Check sheet for the drawn part. Datum: minimum x, y, z corner. Units: mm. Coordinates: 2 decimals unless noted, no trailing zeros. Loops run counter-clockwise (first coordinate to the right, second up) from the corner with the lowest first, then second, coordinate; pieces in that order, holes last. Notation, with made-up numbers: (46.5, -3) - (101.5, -3) arc R19 cw to (101.5, 30) - close; hole circle Ø7 at (-9.5, 33.5). An arc over 180 degrees is marked (long way). Answer as a JSON object with one key per item and string values. Group by question number.
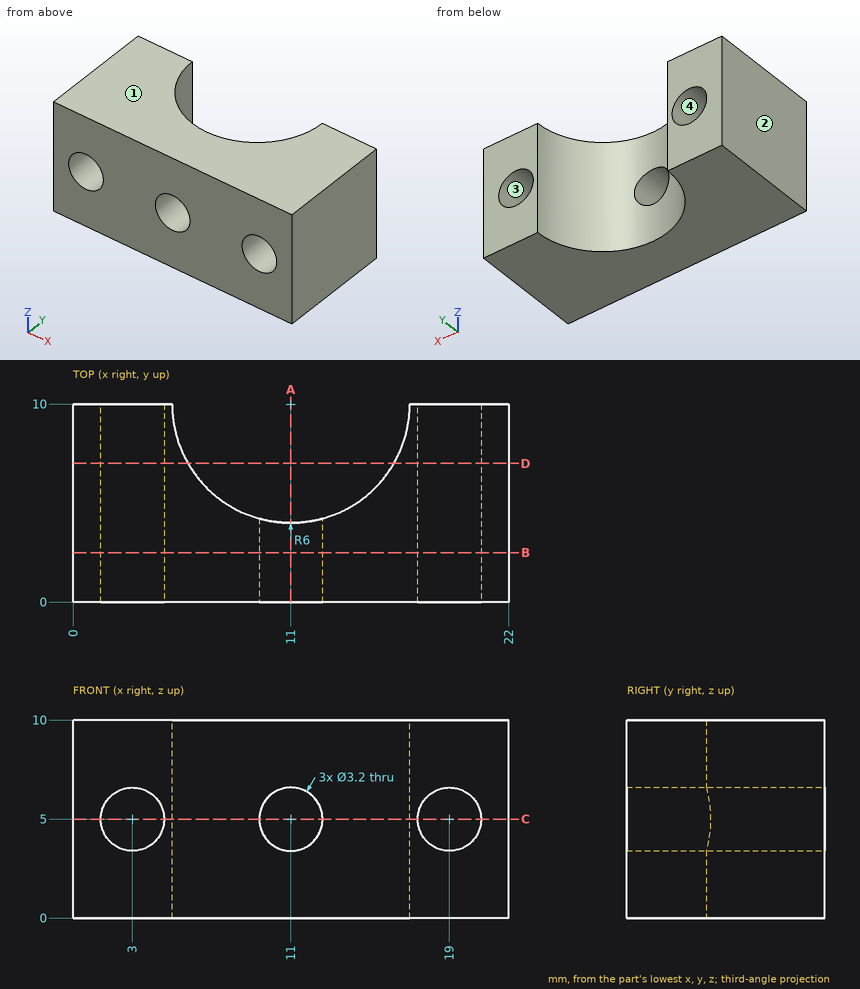
1. Sectioned sample at D-D on y = 7. Record the cut outline in (x, z), plus the area to 4 significant figures.
2. Gauge pin test, flat ends, axial feed: pin 1 (3 mm diameter, centred on x = 12, z = 7, fed in from +Y); pin 2 (1.9 mm diameter, centred on x = 11, z = 5, fed in from +Y). Record the tip position at first contact, or that the pin passes through.
3. Sectioned sample at C-C on z = 5. Record the cut outline in (x, y).
4. Release check for a two-part mould opening along Z. For the marked faces 1, 2, 3 and 4 record: released by +Z, released by -Z, zero draft, split by the parting line, or undercut.
5. Sectioned sample at B-B on y = 2.5. Record the cut outline in (x, z).
6. Sectioned sample at A-A on x = 11. Record the cut outline in (y, z).
7. Material ranges on line 1 (X direction, y = 4.5, z = 4); line 2 (X direction, y = 2.5, z = 5.25); line 3 (Z direction, x = 19, y = 3.5), recorded low to high.
Answers follow:
{
 "1": {"outline": "(0, 0) - (5.8, 0) - (5.8, 10) - (0, 10) - close; (16.2, 0) - (22, 0) - (22, 10) - (16.2, 10) - close; hole circle Ø3.2 at (3, 5); hole circle Ø3.2 at (19, 5)", "area": "100.0 mm^2"},
 "2": {"pin 1": "stops at y = 4.55", "pin 2": "passes through"},
 "3": {"outline": "(0, 0) - (1.4, 0) - (1.4, 10) - (0, 10) - close; (4.6, 0) - (9.4, 0) - (9.4, 4.22) arc R6 cw to (5, 10) - (4.6, 10) - close; (12.6, 0) - (17.4, 0) - (17.4, 10) - (17, 10) arc R6 cw to (12.6, 4.22) - close; (20.6, 0) - (22, 0) - (22, 10) - (20.6, 10) - close"},
 "4": {"face 1": "released by +Z", "face 2": "zero draft", "face 3": "undercut", "face 4": "undercut"},
 "5": {"outline": "(0, 0) - (22, 0) - (22, 10) - (0, 10) - close; hole circle Ø3.2 at (3, 5); hole circle Ø3.2 at (11, 5); hole circle Ø3.2 at (19, 5)"},
 "6": {"outline": "(0, 0) - (4, 0) - (4, 3.4) - (0, 3.4) - close; (0, 6.6) - (4, 6.6) - (4, 10) - (0, 10) - close"},
 "7": {"line 1": "x = 0 to 1.75, 4.25 to 8.6, 13.4 to 17.75, 20.25 to 22", "line 2": "x = 0 to 1.42, 4.58 to 9.42, 12.58 to 17.42, 20.58 to 22", "line 3": "z = 0 to 3.4, 6.6 to 10"}
}
